For this review, use the dimensioned drawing (mm, ordinates from the lowest corner) and the shaded views. Give positions to 0.01 mm unless a question says otherwise; leave off trailing zeros. Loops run counter-clockwise (first coordinate to the right, second up) from the corner with the lowest first, then second, coordinate; pieces in that order, holes last. Notation, with made-up numbers: M -34.75,11.25 L -14.75,11.25 A23 cw -14.75,26.25 Z; hole C -6.75,59.5 d4. An arc over 180 degrees is marked long. Return JSON: item names as keys, results as strings.
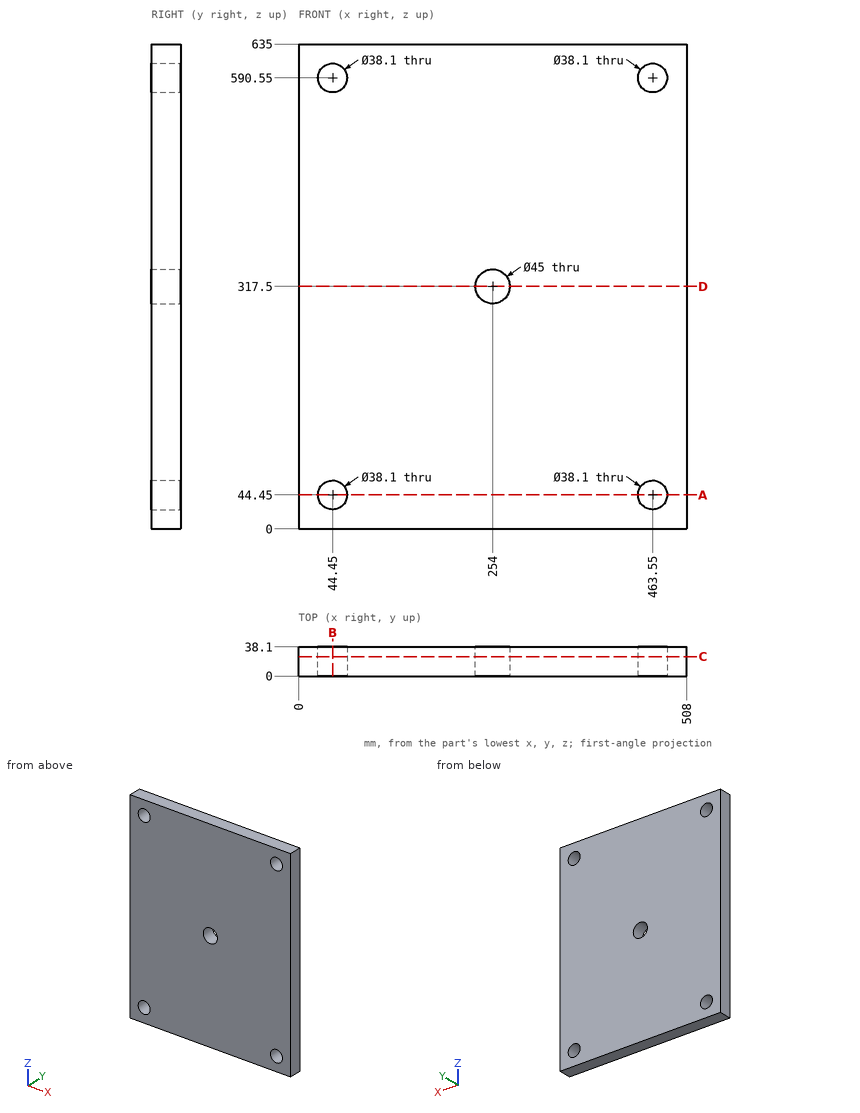
1) Consider section C-C on y = 25.5. Write out the cut boundary in (x, z), then the cut area to 3 significant figures.
From the geometry:
{"outline": "M 0,0 L 508,0 L 508,635 L 0,635 Z; hole C 44.45,44.45 d38.1; hole C 44.45,590.55 d38.1; hole C 254,317.5 d45; hole C 463.55,44.45 d38.1; hole C 463.55,590.55 d38.1", "area": "316,000 mm²"}
2) Consider section B-B on x = 44.45. Write out the cut boundary in (y, z).
From the geometry:
{"outline": "M 0,0 L 38.1,0 L 38.1,25.4 L 0,25.4 Z; M 0,63.5 L 38.1,63.5 L 38.1,571.5 L 0,571.5 Z; M 0,609.6 L 38.1,609.6 L 38.1,635 L 0,635 Z"}
3) Consider section A-A on z = 44.45. Write out the cut boundary in (x, y).
From the geometry:
{"outline": "M 0,0 L 25.4,0 L 25.4,38.1 L 0,38.1 Z; M 63.5,0 L 444.5,0 L 444.5,38.1 L 63.5,38.1 Z; M 482.6,0 L 508,0 L 508,38.1 L 482.6,38.1 Z"}
4) Wall thickness on L1, parallel to Z at x = 44, y = 16; L2, parallel to X at y = 18, z = 590; L3, parallel to Z at x = 46.5, y = 28.5: over which ranges is each line inside the solid? List them lowest first. Write a range as from..to.
From the geometry:
{"L1": "0..25.41, 63.49..571.51, 609.59..635", "L2": "0..25.41, 63.49..444.51, 482.59..508", "L3": "0..25.51, 63.39..571.61, 609.49..635"}
5) Consider section D-D on z = 317.5. Write out the cut boundary in (x, y), then the cut area to 3 significant figures.
From the geometry:
{"outline": "M 0,0 L 231.5,0 L 231.5,38.1 L 0,38.1 Z; M 276.5,0 L 508,0 L 508,38.1 L 276.5,38.1 Z", "area": "17,600 mm²"}
